Autodesk Inventor part; units mm, degrees
ref_plane "YZ Plane" through (0, 0, 0) normal (1, 0, 0) x (0, 1, 0)
ref_plane "XZ Plane" through (0, 0, 0) normal (0, 1, 0) x (-1, 0, 0)
ref_plane "XY Plane" through (0, 0, 0) normal (0, 0, 1) x (1, 0, 0)
sketch "Sketch1" plane through (0, 0, 0) normal (0, 0, 1) x (1, 0, 0)
  circle A0 centre (0, 0) radius 40
  circle A1 centre (0, 0) radius 32.5
  line L0 (0, 0) -> (-26.7142, -26.7142)
  line L1 (0, 0) -> (37.7796, 0) construction
  point P0 (-32.5, 0)
  point P1 (-32.5, 0)
  point P2 (-22.981, -22.981)
  point P3 (-32.5, 0)
  dimension "d0" = 80
  dimension "d1" = 65
  dimension "d3" = 135
extrude "Extrusion1" add sketch "Sketch1" along normal blind 1.2 contours A0 | A1
hole "Hole1" at (-32.5, 0, 0) at (-22.981, -22.981, 0) direction (0, 0, 1) diameter 3 end through all
pattern_circular "Circular Pattern1" count 3 over 360 about axis through (0, 0, -10) along (0, 0, 1) of "Hole1"
properties part number "CNCM_STEEL_Bowl_Electromagnet_Plate" material "Steel"
Model file for the job. Use its own axes, mm. Round coordinates to 2 decimals unless told otherwise and drop trailing zeros. Order: outer loops, then holes, each group sorted by start corner. A loop starts at its lowest first (then second) coordinate and runs counter-clockwise, first axis right, second up.
(1) Pull direction Y, two halves, no side cores. Call faces 1 (the face through (15.236, -29.251, 0.608)), 2 (the face through (-8.67, 39.05, 0.59)), 3 (the face through (-1, 1, 1.2)): released by +Y, released by -Y, zero draft, split by the parting line, or undercut.
(2) Band-saw the part on A-A (y = 0). List the corners of the cut face in (x, z), then the cut area to 3 significant figures.
(3) Band-saw the part on B-B (z = 0.85). List the corners of the cut face in (x, y).
(4) Pin check, flat tip, straight feed: pin 1 (2.5 mm diameter, centred on x = 16.25, y = 28.15, fed in from +Z). Stop position of the tip, or through.
(5) Band-saw the part on D-D (y = 35.5). List the corners of the cut face in (x, z).
(6) Band-saw the part on C-C (x = 16.25). List the corners of the cut face in (y, z), then the cut area to 3 significant figures.
(7) Drill centre lines: line 1 (Y direction, x = 15, z = 0.8); line 2 (Y direction, x = 16, z = 0.8); line 3 (Y direction, x = -32.5, z = 0.9). Where is each one in solid material? Low to high.
Verdict:
1. face 1: undercut
1. face 2: split by the parting line
1. face 3: zero draft
2. outline: (-40, 0) - (-34, 0) - (-34, 1.2) - (-40, 1.2) - close; (-31, 0) - (40, 0) - (40, 1.2) - (-31, 1.2) - close
2. area: 92.4 mm2
3. outline: circle Ø80 at (0, 0); hole circle Ø3 at (-32.5, 0); hole circle Ø3 at (-22.98, -22.98); hole circle Ø3 at (-8.41, 31.39); hole circle Ø3 at (16.25, -28.15); hole circle Ø3 at (16.25, 28.15); hole circle Ø3 at (31.39, -8.41)
4. pin 1: passes through
5. outline: (-18.43, 0) - (18.43, 0) - (18.43, 1.2) - (-18.43, 1.2) - close
6. outline: (-36.55, 0) - (-29.65, 0) - (-29.65, 1.2) - (-36.55, 1.2) - close; (-26.65, 0) - (26.65, 0) - (26.65, 1.2) - (-26.65, 1.2) - close; (29.65, 0) - (36.55, 0) - (36.55, 1.2) - (29.65, 1.2) - close
6. area: 80.5 mm2
7. line 1: y = -37.08 to -28.97, -27.32 to 27.32, 28.97 to 37.08
7. line 2: y = -36.66 to -29.62, -26.67 to 26.67, 29.62 to 36.66
7. line 3: y = -23.32 to -1.5, 1.5 to 23.32
